For this review, take the finished solid that the model builds, in its own axes (mm). Face numbers are marked on the shaded views. A direction names the side the tool comes from. Coordinates: 2 decimals unless noted, no trailing zeros. Order: outer loops, then holes, each group sorted by start corner. A loop starts at its lowest first (then second) coordinate and runs counter-clockwise, first axis right, second up. Notation, with made-up numbers: M 79.25,64.5 L 89.25,64.5 A25 cw 89.25,101.5 Z; hole C 14.5,12.5 d11. An arc over 180 degrees is marked long. Use CSV: the item, a comma, the result in double quotes.
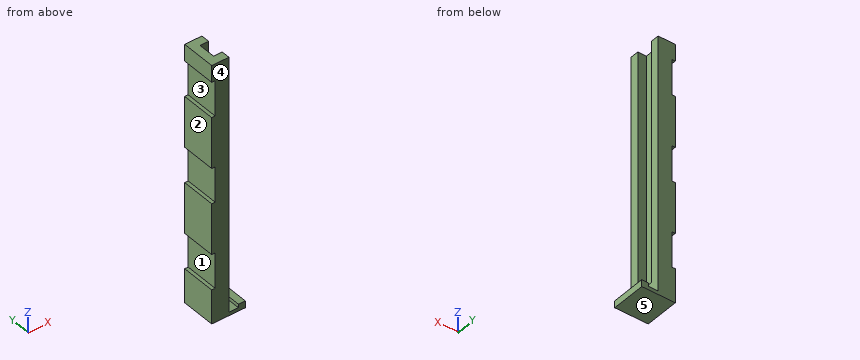
```python
from build123d import *

# Parameters (mm, degrees)
F0_W     = 10
F0_H     = 20
F1_DEPTH = 10
F2_W     = 5.5
F2_H     = 20
F3_DEPTH = 2
F4_W     = 4
F4_H     = 20
F5_DEPTH = 4
F6_W     = 5
F6_H     = 5
F7_DEPTH = 140
F8_W     = 20
F8_H     = 9.75
F8_H_2   = 29.5
F9_DEPTH = 2


with BuildPart() as f1:
    # F0 (on Top) → F1 (new body)
    with BuildSketch(Plane.XY):
        with Locations((5, 10)):
            Rectangle(F0_W, F0_H)
    extrude(amount=F1_DEPTH)

    # F2 (on Top) → F3 (join)
    with BuildSketch(Plane.XY):
        with Locations((12.75, 10)):
            Rectangle(F2_W, F2_H)
    extrude(amount=F3_DEPTH)

    # F4 (on Top) → F5 (join)
    with BuildSketch(Plane.XY):
        with Locations((17.5, 10)):
            Rectangle(F4_W, F4_H)
    extrude(amount=F5_DEPTH)

    # F6 (on face) → F7 (join)
    with BuildSketch(Plane.XY.offset(10)):
        Polygon((5, 20), (2, 20), (2, 0), (5, 0), (5, 5), (5, 15), align=None)
        with Locations((7.5, 17.5)):
            Rectangle(F6_W, F6_H)
        with Locations((7.5, 2.5)):
            Rectangle(F6_W, F6_H)
    extrude(amount=F7_DEPTH)

    # F8 (on face) → F9 (join)
    with BuildSketch(Plane(origin=(2, 0, 0), x_dir=(0, -1, 0), z_dir=(-1, 0, 0))):
        with Locations((-10, 145.125)):
            Rectangle(F8_W, F8_H)
        with Locations((-10, 105)):
            Rectangle(F8_W, F8_H_2)
        with Locations((-10, 55)):
            Rectangle(F8_W, F8_H_2)
        with Locations((-10, 14.875)):
            Rectangle(F8_W, F8_H)
    extrude(amount=F9_DEPTH)


solid = f1.part
```
Item 1: Draft analysis for pull direction Z (two halves, no side actions). For the marked faces 3, 4 and 5, state which applies: released by +Z, released by -Z, zero draft, split by the parting line, or undercut.
Solutions:
face 3,"undercut"
face 4,"zero draft"
face 5,"released by -Z"
Item 2: Clearance check with flat-ended pins moving along their axes: pin 1 Ø6 at (y, z) = (11.5, 46) entering from +X; pin 2 Ø10 at (y, z) = (7.5, 133) entering from -X; pin 3 Ø2 at (x, y) = (17, 15) entering from +Z. State where each tip first meets the part, or that it passes through.
Solutions:
pin 1,"x = 5"
pin 2,"x = 2"
pin 3,"z = 4"
Item 3: Add section A-A on x = 6.75. State the section outline as (y, z) points.
Solutions:
outline,"M 0,0 L 20,0 L 20,150 L 15,150 L 15,10 L 5,10 L 5,150 L 0,150 Z"
Item 4: Add section B-B on z = 131. State the section outline as (x, y) points.
Solutions:
outline,"M 2,0 L 10,0 L 10,5 L 5,5 L 5,15 L 10,15 L 10,20 L 2,20 Z"
Item 5: Add section D-D on x = 13.5. State the section outline as (y, z) points, and give its area (3 significant figures).
Solutions:
outline,"M 0,0 L 20,0 L 20,2 L 0,2 Z"
area,"40.0 mm^2"
Item 6: For the marked faces 1 and 2, list the 3-axis set-ups (+Z, -Z, +X, -X, +Y, -Y) from which the entire face can be reached by the end or side of a thin tool; tool diameter is ignored.
Solutions:
face 1,"-X, +Y, -Y"
face 2,"+Z, -Z, -X, +Y, -Y"
Item 7: Add section C-C on y = 10.5. State the section outline as (x, z) points.
Solutions:
outline,"M 0,0 L 19.5,0 L 19.5,4 L 15.5,4 L 15.5,2 L 10,2 L 10,10 L 5,10 L 5,150 L 0,150 L 0,140.25 L 2,140.25 L 2,119.75 L 0,119.75 L 0,90.25 L 2,90.25 L 2,69.75 L 0,69.75 L 0,40.25 L 2,40.25 L 2,19.75 L 0,19.75 Z"
Item 8: To check wall thickness, follow line 1 along Z through (x, y) = (1, 11.75); line 2 along Y through (x, z) = (6, 39); line 3 along X through (y, z) = (14, 113.5). State the ranges of each line that lie inside material, in increasing order. Write a range as [from, to].
Solutions:
line 1,"[0, 19.75], [40.25, 69.75], [90.25, 119.75], [140.25, 150]"
line 2,"[0, 5], [15, 20]"
line 3,"[0, 5]"
